Here's how the part is built. I have some questions about the finished solid (model axes, mm). Face numbers are marked on the shaded views. A direction names the side the tool comes from. Give positions to 0.01 mm unless a question says otherwise; leave off trailing zeros. Write each loop counter-clockwise with the first axis right and the second up, starting at its lowest first coordinate (ties: lowest second). Pieces come first, ordered by that corner, then holes. Notation, with made-up numbers: (19.25, -12) -> (53.25, -12) arc R20 ccw to (53.25, 25) -> close; hole circle Ø11 at (-9, 25.25). An arc over 180 degrees is marked (long way). Return JSON: item names as keys, results as strings.
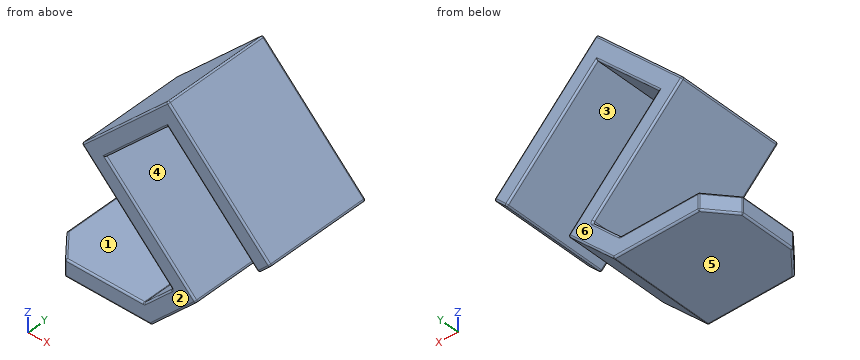
from build123d import *

# Parameters (mm, degrees)
PAD_DEPTH    = 4
PAD001_DEPTH = 25
FILLET_R     = 0.4


with BuildPart() as part:
    # Sketch → Pad (new body)
    with BuildSketch(Plane.XY):
        Polygon((5, 0), (0, 5.958768), (0, 19.041232), (5, 25), (25, 25), (25, 0), align=None)
    extrude(amount=PAD_DEPTH)

    # Sketch001 → Pad001 (join)
    with BuildSketch(Plane.XZ):
        Polygon((29.949747, 10.606602), (19.343146, 0), (25, 0), (35.606602, 10.606602), (14.393398, 31.819805), (28.889087, 46.315494), (50.102291, 25.102291), (52.930718, 27.930718), (28.889087, 51.972348), (8.736544, 31.819805), align=None)
    extrude(amount=-PAD001_DEPTH)

    # Fillet
    fillet_edges = [part.edges().sort_by_distance(p)[0] for p in [
        (25, 0, 21.213203),
        (21.641243, 0, 39.06765),
        (18.812816, 0, 41.896077),
        (19.343146, 0, 21.213203),
        (26.646447, 0, 7.303301),
        (30.303301, 0, 5.303301),
        (12.171573, 0, 0),
        (22.171573, 0, 0),
        (14.171573, 0, 4),
        (2.5, 2.979384, 4),
        (2.5, 2.979384, 0),
        (5, 0, 2),
        (0, 5.958768, 2),
        (39.495689, 0, 35.708892),
        (40.909903, 0, 39.951533),
        (50.102291, 12.5, 25.102291),
        (51.516504, 0, 26.516504),
        (8.736544, 12.5, 31.819805),
        (0, 12.5, 4),
        (0, 12.5, 0),
        (0, 19.041232, 2),
        (2.5, 22.020616, 4),
        (2.5, 22.020616, 0),
        (5, 25, 2),
        (18.812816, 25, 41.896077),
        (28.889087, 12.5, 51.972348),
        (19.343146, 25, 21.213203),
        (29.949747, 12.5, 10.606602),
        (23.343146, 12.5, 4),
        (14.171573, 25, 4),
        (12.171573, 25, 0),
        (22.171573, 25, 0),
        (30.303301, 25, 5.303301),
        (25, 25, 21.213203),
        (21.641243, 25, 39.06765),
        (39.495689, 25, 35.708892),
        (40.909903, 25, 39.951533),
        (51.516504, 25, 26.516504),
        (52.930718, 12.5, 27.930718),
        (35.606602, 12.5, 10.606602),
        (26.646447, 25, 7.303301),
        (25, 12.5, 0),
    ]]
    fillet(fillet_edges, radius=FILLET_R)


solid = part.part
1. Suppose I cut it at B-B, the plane x = 22. Count the separate pieces of the cut face and the enclosed holes in it, and give its area (3 significant figures).
Taken from the geometry:
{"separate pieces": "3", "enclosed holes": "0", "area": "382 mm²"}
2. If we mould it in two halves opening along Z, with no side actions, what happens to the marked faces 4, 5 and 6? For each: released by +Z, released by -Z, zero draft, split by the parting line, or undercut.
Taken from the geometry:
{"face 4": "undercut", "face 5": "released by -Z", "face 6": "zero draft"}
3. For pin 1 Ø1.5 at (x, y) = (42, 15.5) entering from +Z; pin 2 Ø1 at (y, z) = (20, 29.5) entering from -X; pin 3 Ø5 at (y, z) = (5, 17.5) entering from -X, each with a flat end and sliding along its axis, tell me the tip position at first contact or that it passes through.
Taken from the geometry:
{"pin 1": "stops at z = 39.61", "pin 2": "stops at x = 10.56", "pin 3": "stops at x = 20.56"}
4. Which directions (+Z, -Z, +X, -X, +Y, -Y) give clear straight access to the entire face, cutting with the end or side of a thin tool? Please do the marked faces 1, 2 and 3.
Taken from the geometry:
{"face 1": "-X, +Y, -Y", "face 2": "+Z, -Z, +X, -X, -Y", "face 3": "+Y, -Y"}
5. Suppose I cut it at A-A, the plane y = 8.25. List the corners of the cut face in (x, z) for me, and give its area (3 significant figures).
Taken from the geometry:
{"outline": "(0, 0.4) arc R0.4 ccw to (0.4, 0) -> (24.83, 0) arc R0.4 ccw to (25.12, 0.12) -> (35.32, 10.32) arc R0.4 ccw to (35.32, 10.89) -> (14.39, 31.82) -> (28.89, 46.32) -> (49.82, 25.39) arc R0.4 ccw to (50.39, 25.39) -> (52.65, 27.65) arc R0.4 ccw to (52.65, 28.21) -> (29.17, 51.69) arc R0.4 ccw to (28.61, 51.69) -> (9.02, 32.1) arc R0.4 ccw to (9.02, 31.54) -> (29.67, 10.89) arc R0.4 cw to (29.67, 10.32) -> (23.46, 4.12) arc R0.4 cw to (23.18, 4) -> (0.4, 4) arc R0.4 ccw to (0, 3.6) -> close", "area": "491 mm²"}
6. If I drill on line 1 (Z direction, x = 17.5, y = 15); line 2 (Z direction, x = 25, y = 13.75); line 3 (X direction, y = 10.5, z = 39), over which ranges is the centre line in solid material (lowest first)? Write a range as [from, to].
Taken from the geometry:
{"line 1": "z = [0, 4], [23.06, 28.71], [34.93, 40.58]", "line 2": "z = [0.04, 5.66], [15.56, 21.21], [42.43, 48.08]", "line 3": "x = [15.92, 21.57], [36.2, 41.86]"}
